Part print with two shaded views. Sizes in mm from the minimum x, y, z corner. A direction names the side the tool comes from. Round coordinates to 2 decimals unless told otherwise and drop trailing zeros. Order: outer loops, then holes, each group sorted by start corner. A loop starts at its lowest first (then second) coordinate and runs counter-clockwise, first axis right, second up. Notation, with made-up numbers: M -19,10 L 3,10 A14 ccw 3,14 Z; hole C 79.5,-3.75 d3. An arc over 180 degrees is marked long. Put each result on its own line as item: value.
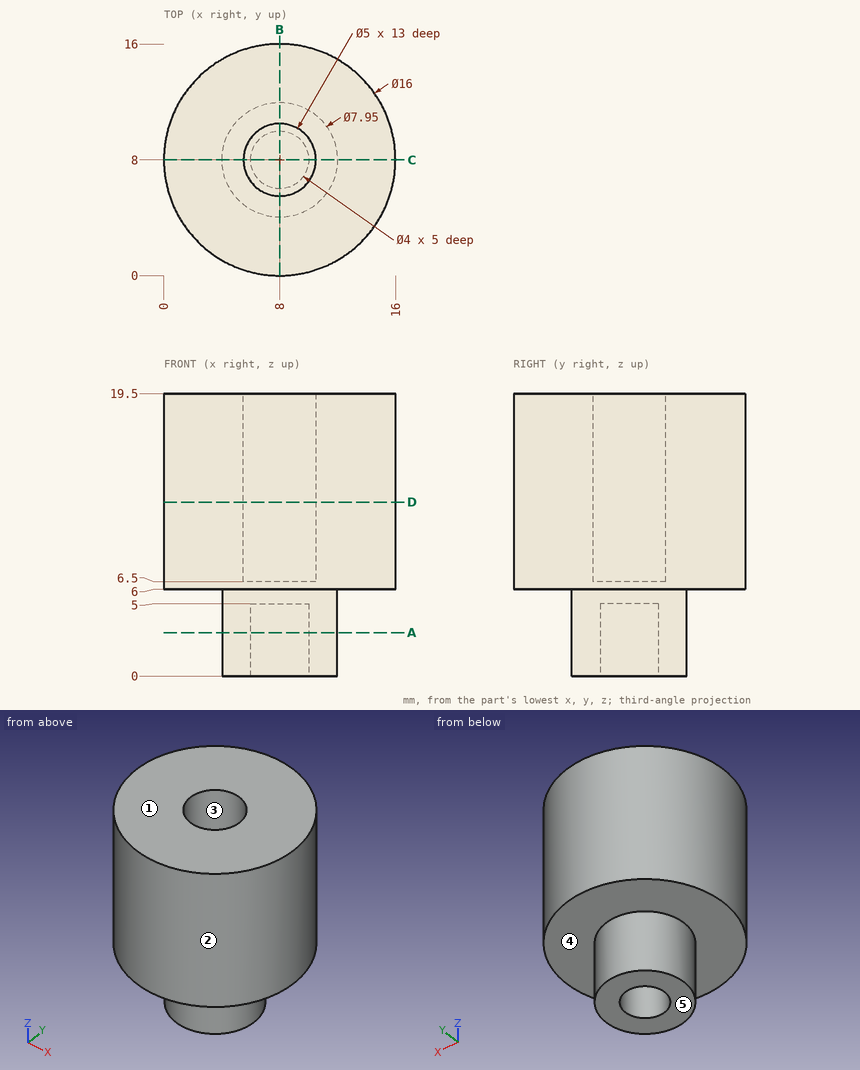
Item 1: Pin check, flat tips, straight feed: P1, Ø2, axis at x = 10, z = 15, coming from the +Y side; P2, Ø6, axis at x = 11.5, z = 14, coming from the -Y side; P3, Ø6, axis at x = 11.5, y = 6.5, coming from the -Z side; P4, Ø1.5, axis at x = 5.5, z = 6, coming from the -Y side. Stop position of each tip, or through.
Answers below:
P1: y = 15.94
P2: y = 0.02
P3: z = 0
P4: y = 0.19
Item 2: Mould opens along Y. For the marked faces 1, 2 and 3 say: pulls with the +Y half, pulls with the -Y half, needs draft (parallel to the pull), parting line crosses it, or undercut.
Answers below:
face 1: needs draft
face 2: parting line crosses it
face 3: undercut
Item 3: Probe line 1 along Y through (x, z) = (8, 10.25); line 2 along Y through (x, z) = (8, 2.4) (3 decimals); line 3 along Z through (x, y) = (13.75, 9). List the from-to ranges inside material, lowest first. Write a range as [from, to].
Answers below:
line 1: [0, 5.5], [10.5, 16]
line 2: [4.025, 6], [10, 11.975]
line 3: [6, 19.5]
Item 4: Band-saw the part on A-A on z = 3. Give the cut face in (x, y) (3 decimals).
Answers below:
outline: C 8,8 d7.95; hole C 8,8 d4
Item 5: Band-saw the part on B-B on x = 8. Give the cut face in (y, z) (3 decimals), and give its area (3 significant figures).
Answers below:
outline: M 0,6 L 4.025,6 L 4.025,0 L 6,0 L 6,5 L 10,5 L 10,0 L 11.975,0 L 11.975,6 L 16,6 L 16,19.5 L 10.5,19.5 L 10.5,6.5 L 5.5,6.5 L 5.5,19.5 L 0,19.5 Z
area: 179 mm²
Item 6: Tool access for the marked faces 4 and 5: list every direction of +Z, -Z, +X, -X, +Y, -Y with a clear straight run to the whole face (end or side of a thin tool).
Answers below:
face 4: -Z
face 5: -Z, +X, -X, +Y, -Y
Item 7: Band-saw the part on D-D on z = 12. Give the cut face in (x, y).
Answers below:
outline: C 8,8 d16; hole C 8,8 d5
